from build123d import *

# Parameters (mm, degrees)
SKETCH1_R           = 11
SKETCH1_R_2         = 7.5
EXTRUDE_THIN1_DEPTH = 5
BOSS_EXTRUDE2_DEPTH = 5
SKETCH4_W           = 5
SKETCH4_H           = 3
BOSS_EXTRUDE3_DEPTH = 10
SKETCH5_R           = 1
CUT_EXTRUDE1_DEPTH  = 5
LPATTERN1_COUNT     = 2
LPATTERN1_PITCH     = 32
SKETCH6_W           = 10
SKETCH6_H           = 6.354024863
CUT_EXTRUDE2_DEPTH  = 5


with BuildPart() as part:
    # Sketch1 → Extrude-Thin1 (new body)
    with BuildSketch(Plane(origin=(0, 0, 0), x_dir=(0, 0, -1), z_dir=(1, 0, 0))):
        Circle(SKETCH1_R)
        Circle(SKETCH1_R_2, mode=Mode.SUBTRACT)
    extrude(amount=EXTRUDE_THIN1_DEPTH)

    # Sketch2 → Boss-Extrude2 (add)
    with BuildSketch(Plane(origin=(0, 0, 0), x_dir=(0, 0, -1), z_dir=(1, 0, 0))):
        with BuildLine():
            Line((-11, 0), (-11, 25))
            Line((-11, 25), (11, 25))
            Line((11, 25), (11, 0))
            ThreePointArc((11, 0), (0, 11), (-11, 0))
        make_face()
    extrude(amount=BOSS_EXTRUDE2_DEPTH)

    # Sketch4 → Boss-Extrude3 (add)
    with BuildSketch(Plane(origin=(0, 0, -11), x_dir=(-1, 0, 0), z_dir=(0, 0, -1))):
        with Locations((-2.5, 23.5)):
            Rectangle(SKETCH4_W, SKETCH4_H)
    boss_extrude3 = extrude(amount=BOSS_EXTRUDE3_DEPTH)

    # Sketch5 → Cut-Extrude1 (cut)
    with BuildSketch(Plane(origin=(0, 25, 0), x_dir=(1, 0, 0), z_dir=(0, 1, 0))):
        with Locations(Location((2.5, 16, 0), (0, 0, 270))):
            Circle(SKETCH5_R)
    cut_extrude1 = extrude(amount=-CUT_EXTRUDE1_DEPTH, mode=Mode.SUBTRACT)

    # LPattern1: Boss-Extrude3, Cut-Extrude1 ×2
    with Locations(*[(0, 0, i * LPATTERN1_PITCH) for i in range(1, LPATTERN1_COUNT)]):
        add(boss_extrude3)
        add(cut_extrude1, mode=Mode.SUBTRACT)

    # Sketch6 → Cut-Extrude2 (cut)
    with BuildSketch(Plane(origin=(5, 0, 0), x_dir=(0, 0, -1), z_dir=(1, 0, 0))):
        with Locations((0, 15.177012432)):
            Rectangle(SKETCH6_W, SKETCH6_H)
    extrude(amount=-CUT_EXTRUDE2_DEPTH, mode=Mode.SUBTRACT)


solid = part.part
Source: CAD feature listing. Evaluate the final solid. Frame: model axes, mm. A direction names the side the tool comes from. Round coordinates to 2 decimals unless told otherwise and drop trailing zeros. Loops run counter-clockwise (first coordinate to the right, second up) from the corner with the lowest first, then second, coordinate; pieces in that order, holes last. Notation, with made-up numbers: (69, -13) -> (84, -13) arc R19 cw to (84, 0) -> close; hole circle Ø10 at (60.5, 4). An arc over 180 degrees is marked (long way). Answer as a JSON object with one key per item and string values. Group by question number.
Q1. Section query D-D (z = 0). Output: boundary loops of the cut face in (x, y).
Q2. Contact query for flat-ended pins moving along their axis: P1, Ø1.5, axis at x = 3.5, z = -17, coming from the -Y side; P2, Ø1.5, axis at x = 3.5, y = 7.5, coming from the +Z side. Output: stop coordinate, or through.
Q3. Mould query, pull axis X, two halves, no side actions, for faces 4 (the flat face through (0, 11, 0)), 5 (the flat face through (1, 22, -16)), 6 (the cylindrical face through (2.8, 23.521, 16.954)). Classes: pulls with the +X half, pulls with the -X half, needs draft (parallel to the pull), parting line crosses it, or undercut.
Q4. Section query C-C (z = -16). Output: boundary loops of the cut face in (x, y), plus the area to 3 significant figures.
Q5. Access query for faces 1 (the flat face through (2, 11, -11)), 2 (the flat face through (3, 18.354, 0)), 3 (the flat face through (2, 11, 11)). Directions: +Z, -Z, +X, -X, +Y, -Y. A direction counts if a zero-diameter tool reaches every point of the face in a straight line with its end or side. Return the directions, or none.
Q6. Section query A-A (x = 2.5). Output: boundary loops of the cut face in (y, z).
Q7. Ray query, line 1 (Y direction, x = 2.6, z = 0); line 2 (Z direction, x = 3.4, y = 15.5); line 3 (X direction, y = 23.1, z = 16). Return the intervals inside material, ascending. Write a range as from..to.
Q8. Section query B-B (y = 17.5). Output: boundary loops of the cut face in (x, z).
Completed:
{
 "1": {"outline": "(0, -11) -> (5, -11) -> (5, -7.5) -> (0, -7.5) -> close; (0, 7.5) -> (5, 7.5) -> (5, 12) -> (0, 12) -> close; (0, 18.35) -> (5, 18.35) -> (5, 25) -> (0, 25) -> close"},
 "2": {"P1": "y = 22", "P2": "z = 11"},
 "3": {"face 4": "pulls with the -X half", "face 5": "needs draft", "face 6": "undercut"},
 "4": {"outline": "(0, 22) -> (1.5, 22) -> (1.5, 25) -> (0, 25) -> close; (3.5, 22) -> (5, 22) -> (5, 25) -> (3.5, 25) -> close", "area": "9.00 mm²"},
 "5": {"face 1": "-Z, +X, -X, -Y", "face 2": "+X, -X", "face 3": "+Z, +X, -X, -Y"},
 "6": {"outline": "(0, -11) -> (22, -11) -> (22, -15) -> (25, -15) -> (25, 15) -> (22, 15) -> (22, 11) -> (0, 11) arc R11 ccw to start; (22, -21) -> (25, -21) -> (25, -17) -> (22, -17) -> close; (22, 17) -> (25, 17) -> (25, 21) -> (22, 21) -> close; hole circle Ø15 at (0, 0); hole (12, -5) -> (18.35, -5) -> (18.35, 5) -> (12, 5) -> close"},
 "7": {"line 1": "-11..-7.5, 7.5..12, 18.35..25", "line 2": "-11..-5, 5..11", "line 3": "0..1.5, 3.5..5"},
 "8": {"outline": "(0, -11) -> (5, -11) -> (5, -5) -> (0, -5) -> close; (0, 5) -> (5, 5) -> (5, 11) -> (0, 11) -> close"}
}
